Print and shaded views of the part. All mm, measured from the part's lowest x, y and z. A direction names the side the tool comes from. Give positions to 0.01 mm unless a question says otherwise; leave off trailing zeros. Order: outer loops, then holes, each group sorted by start corner. A loop starts at its lowest first (then second) coordinate and runs counter-clockwise, first axis right, second up. Notation, with made-up numbers: (-14, 62) - (25, 62) arc R20 ccw to (25, 93) - close; hole circle Ø11 at (62.5, 73). An arc over 180 degrees is marked (long way). Answer in a Markdown table with one row per item.
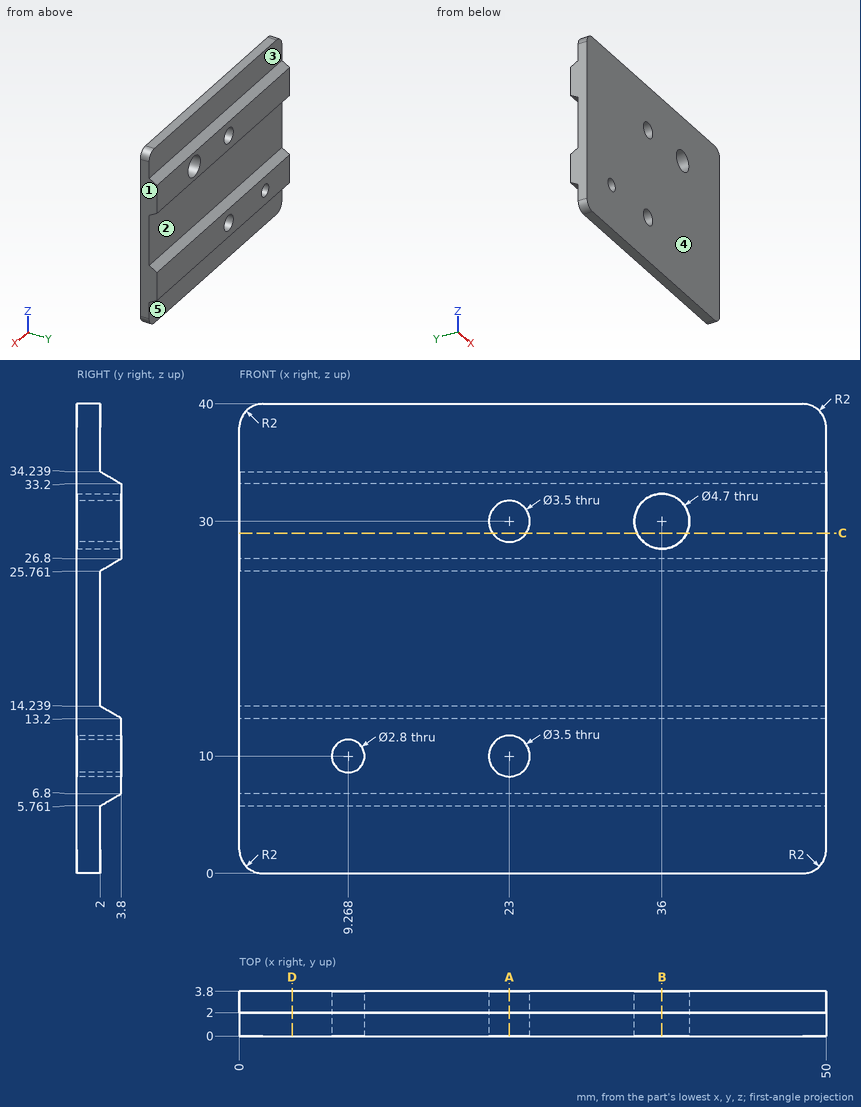
1. Two-plate mould, pull along Z, no slides. Class the marked faces 1 and 2: +Z half, -Z half, draft (parallel to the pull), parting line (faces both ways), or undercut.
Check result:
| item | result |
|---|---|
| face 1 | draft |
| face 2 | undercut |
2. Cut at B-B on x = 36. Write the cut outline in (y, z).
Check result:
| item | result |
|---|---|
| outline | (0, 0) - (2, 0) - (2, 5.76) - (3.8, 6.8) - (3.8, 13.2) - (2, 14.24) - (2, 25.76) - (3.8, 26.8) - (3.8, 27.65) - (0, 27.65) - close; (0, 32.35) - (3.8, 32.35) - (3.8, 33.2) - (2, 34.24) - (2, 40) - (0, 40) - close |
3. Probe line 1 (Z direction, x = 23, y = 1.75); line 2 (X direction, y = 1.35, z = 29); line 3 (Z direction, x = 36, y = 1.1). List the from-to ranges inside material, lowest first.
Check result:
| item | result |
|---|---|
| line 1 | z = 0 to 8.25, 11.75 to 28.25, 31.75 to 40 |
| line 2 | x = 0 to 21.56, 24.44 to 33.87, 38.13 to 50 |
| line 3 | z = 0 to 27.65, 32.35 to 40 |
4. Which spindle directions (+Z, -Z, +X, -X, +Y, -Y) get a long thin tool onto all of the face, cutting with end or side? Do the marked faces 3, 4 and 5. Say none if no direction does.
Check result:
| item | result |
|---|---|
| face 3 | +Z, +X, -X, +Y |
| face 4 | +Z, -Z, +X, -X, -Y |
| face 5 | -Z, +X, -X, +Y |
5. Cut at D-D on x = 4.5. Write the cut outline in (y, z).
Check result:
| item | result |
|---|---|
| outline | (0, 0) - (2, 0) - (2, 5.76) - (3.8, 6.8) - (3.8, 13.2) - (2, 14.24) - (2, 25.76) - (3.8, 26.8) - (3.8, 33.2) - (2, 34.24) - (2, 40) - (0, 40) - close |
6. Cut at C-C on z = 29. Write the cut outline in (x, y).
Check result:
| item | result |
|---|---|
| outline | (0, 0) - (21.56, 0) - (21.56, 3.8) - (0, 3.8) - close; (24.44, 0) - (33.87, 0) - (33.87, 3.8) - (24.44, 3.8) - close; (38.13, 0) - (50, 0) - (50, 3.8) - (38.13, 3.8) - close |
7. Cut at A-A on x = 23. Write the cut outline in (y, z).
Check result:
| item | result |
|---|---|
| outline | (0, 0) - (2, 0) - (2, 5.76) - (3.8, 6.8) - (3.8, 8.25) - (0, 8.25) - close; (0, 11.75) - (3.8, 11.75) - (3.8, 13.2) - (2, 14.24) - (2, 25.76) - (3.8, 26.8) - (3.8, 28.25) - (0, 28.25) - close; (0, 31.75) - (3.8, 31.75) - (3.8, 33.2) - (2, 34.24) - (2, 40) - (0, 40) - close |
8. Drop flat-ended pins along their axis: P1, Ø9, axis at x = 22, z = 18.5, coming from the +Y side (1 decimal); P2, Ø1.7, axis at x = 33.5, z = 2, coming from the +Y side; P3, Ø4, axis at x = 23, z = 30, coming from the +Y side. Give the stop position or say it passes through.
Check result:
| item | result |
|---|---|
| P1 | stops at y = 2.4 |
| P2 | stops at y = 2 |
| P3 | stops at y = 3.8 |
